For this review, take the finished solid that the model builds, in its own axes (mm). A direction names the side the tool comes from. Give positions to 0.01 mm unless a question says otherwise; leave off trailing zeros. Order: outer loops, then holes, each group sorted by start corner. A loop starts at its lowest first (then second) coordinate and runs counter-clockwise, first axis right, second up. Notation, with made-up numbers: (82.5, 31) - (141.5, 31) arc R37 ccw to (141.5, 67) - close; hole circle Ø8 at (58, 51.25). An arc over 180 degrees is marked (long way). Answer as a JSON object with one key per item and string values. Group by question number.
from build123d import *

# Parameters (mm, degrees)
SKETCH1_R                      = 3.7
BOSS_EXTRUDE1_DEPTH            = 109
F_4_0MM_DOWEL_HOLE1_AT_2_COUNT = 2
F_4_0MM_DOWEL_HOLE1_AT_2_PITCH = 98.7
F_4_0MM_DOWEL_HOLE2_AT_2_COUNT = 2
F_4_0MM_DOWEL_HOLE2_AT_2_PITCH = 98.7
SKETCH7_W                      = 0.2
SKETCH7_H                      = 7
CHAMFER1_SIZE                  = 0.2
CUT_EXTRUDE2_DEPTH             = 110.139452178
CUT_EXTRUDE2_DEPTH_BACK        = 110.139452178
SKETCH8_R                      = 1.3


with BuildPart() as part:
    # Sketch1 → Boss-Extrude1 (new body)
    with BuildSketch(Plane(origin=(0, 0, 0), x_dir=(1, 0, 0), z_dir=(0, 1, 0))):
        with Locations(Location((0, 0, 0), (0, 0, 270))):
            Circle(SKETCH1_R)
    extrude(amount=BOSS_EXTRUDE1_DEPTH)

    # Sketch4 → Ø4.0mm Dowel Hole1 (revolve, cut)
    with BuildSketch(Plane(origin=(0, 5.15, 0), x_dir=(0, 0, -1), z_dir=(0, 1, 0))):
        Polygon((0, 0), (0, 3.7), (2, 3.7), (2, 0.025), (2.025, 0), align=None)
    f_4_0mm_dowel_hole1 = revolve(axis=Axis((6.35, 5.15, 0), (-1, 0, 0)), mode=Mode.SUBTRACT)

    # Ø4.0mm Dowel Hole1 at 2: Ø4.0mm Dowel Hole1 ×2
    with Locations(*[(0, i * F_4_0MM_DOWEL_HOLE1_AT_2_PITCH, 0) for i in range(1, F_4_0MM_DOWEL_HOLE1_AT_2_COUNT)]):
        add(f_4_0mm_dowel_hole1, mode=Mode.SUBTRACT)

    # Sketch6 → Ø4.0mm Dowel Hole2 (revolve, cut)
    with BuildSketch(Plane.ZX.offset(103.85)):
        Polygon((0, 0), (0, 3.7), (2, 3.7), (2, 0.025), (2.025, 0), align=None)
    f_4_0mm_dowel_hole2 = revolve(axis=Axis((-6.35, 103.85, 0), (1, 0, 0)), mode=Mode.SUBTRACT)

    # Ø4.0mm Dowel Hole2 at 2: Ø4.0mm Dowel Hole2 ×2
    with Locations(*[(0, -i * F_4_0MM_DOWEL_HOLE2_AT_2_PITCH, 0) for i in range(1, F_4_0MM_DOWEL_HOLE2_AT_2_COUNT)]):
        add(f_4_0mm_dowel_hole2, mode=Mode.SUBTRACT)

    # Sketch7 → Revolve1 (revolve)
    with BuildSketch(Plane(origin=(0, 0, 0), x_dir=(0, 0, -1), z_dir=(1, 0, 0)), mode=Mode.PRIVATE) as revolve1_sk:
        with Locations((3.8, 93.5)):
            Rectangle(SKETCH7_W, SKETCH7_H)
        with Locations((3.8, 15.5)):
            Rectangle(SKETCH7_W, SKETCH7_H)
    revolve(revolve1_sk.sketch.rotate(Axis((0, 99.222233113, 0), (0, -1, 0)), 180), axis=Axis((0, 99.222233113, 0), (0, -1, 0)))

    # Chamfer1
    chamfer1_edges = [part.edges().sort_by_distance(p)[0] for p in [
        (0, 97, -3.7),
        (0, 90, -3.7),
        (0, 19, -3.7),
        (0, 12, -3.7),
    ]]
    chamfer(chamfer1_edges, length=CHAMFER1_SIZE - 0.0001)  # a hair under: the kernel refuses the full size

    # Sketch8 → Cut-Extrude2 (cut, two sides: drawn at the far end of the back side and taken through both)
    with BuildSketch(Plane(origin=(0, 0, 0), x_dir=(0, 0, -1), z_dir=(1, 0, 0)).offset(-CUT_EXTRUDE2_DEPTH_BACK)):
        with Locations((0, 66)):
            Circle(SKETCH8_R)
    extrude(amount=CUT_EXTRUDE2_DEPTH + CUT_EXTRUDE2_DEPTH_BACK, mode=Mode.SUBTRACT)


solid = part.part
1) Mouldability with a two-part tool opening along Z and no side actions: class faces 1 (the face through (2.5, 5.82, -2.73)), 2 (the face through (0, 109, 0)), 3 (the face through (-1.837, 104.616, -1.847)), 4 (the face through (-0.05, 64.73, 0.28)) as released by +Z, released by -Z, zero draft, split by the parting line, or undercut.
2) Consider section A-A (y = 103.85). Give the boundary of the cut face in (x, z) (3 decimals), plus the area to 3 significant figures.
3) For line 1 (Y direction, x = 0, z = 0) (3 decimals); line 2 (Y direction, x = 1.4, z = 0); line 3 (Y direction, x = -2.5, z = -1.5), list the stretches that pass through material, from the lowest coordinate up.
4) Consider section B-B (z = 0). Give the number of separate pieces and of enclosed holes in the cut face, plus the area to 3 significant figures.
5) For pin 1 (3 mm diameter, centred on y = 84, z = 1.5, fed in from -X); pin 2 (3 mm diameter, centred on y = 103.85, z = 0, fed in from +X); pin 3 (4 mm diameter, centred on y = 63.5, z = -1.5, fed in from +X), all flat-tipped, find the tip position at first contact; note any pin that passes through.
6) Consider section C-C (y = 30). Give the boundary of the cut face in (x, z).
7) For faces 5 (the face through (-1.837, 5.916, -1.847)), 6 (the face through (-3.612, 54.006, -0.802)), 7 (the face through (3.12, 103.02, 1.99)), list the 3-axis set-ups (+Z, -Z, +X, -X, +Y, -Y) from which the entire face can be reached by the end or side of a thin tool; tool diameter is ignored.
Result set:
{
 "1": {"face 1": "split by the parting line", "face 2": "zero draft", "face 3": "undercut", "face 4": "undercut"},
 "2": {"outline": "(-3.113, -2) arc R3.7 ccw to (3.113, -2) - (0.025, -2) - (0, -2.025) - (-0.025, -2) - close; (-3.113, 2) - (-0.025, 2) - (0, 2.025) - (0.025, 2) - (3.113, 2) arc R3.7 ccw to start", "area": "14.9 mm2"},
 "3": {"line 1": "y = 0 to 3.125, 7.175 to 64.7, 67.3 to 101.825, 105.875 to 109", "line 2": "y = 0 to 3.15, 7.15 to 64.7, 67.3 to 101.85, 105.85 to 109", "line 3": "y = 0 to 3.83, 6.47 to 102.53, 105.17 to 109"},
 "4": {"separate pieces": "4", "enclosed holes": "0", "area": "734 mm2"},
 "5": {"pin 1": "stops at x = -3.7", "pin 2": "passes through", "pin 3": "stops at x = 3.7"},
 "6": {"outline": "circle Ø7.4 at (0, 0)"},
 "7": {"face 5": "+X, -X", "face 6": "none", "face 7": "+Y"}
}
